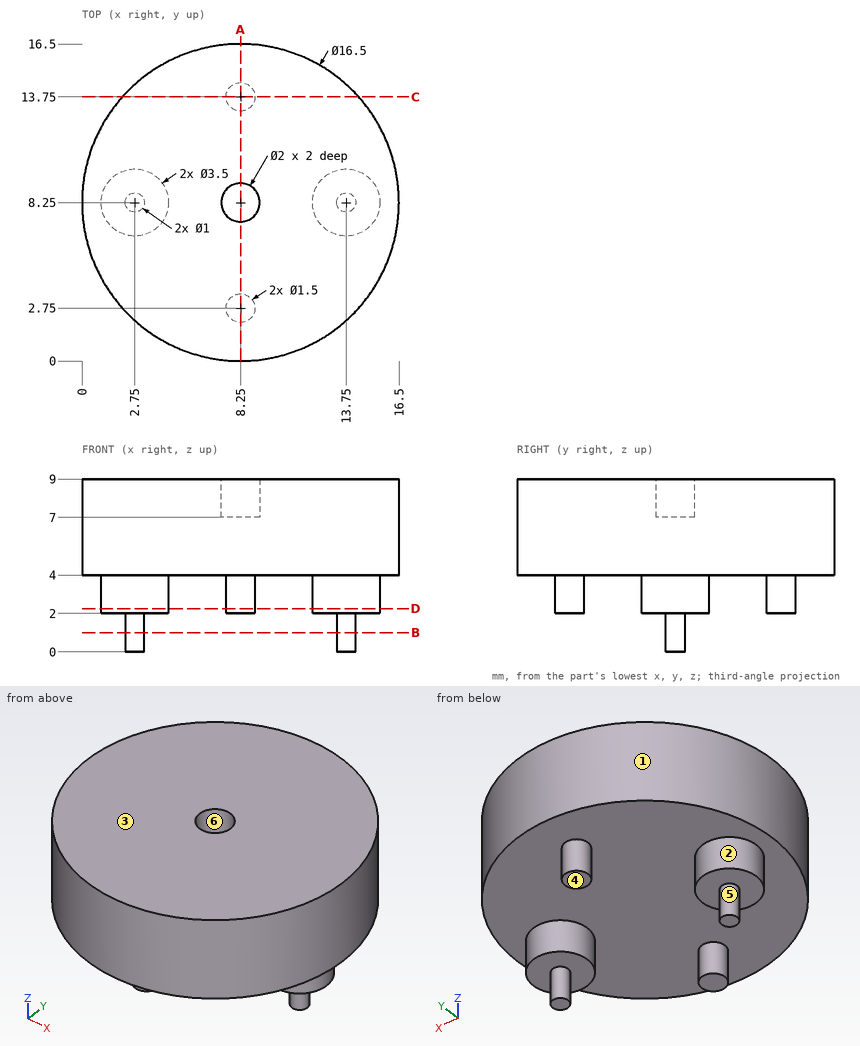
Input: dimensioned drawing with shaded views. Units: mm. Origin: part minimum x, y, z. A direction names the side the tool comes from. Coordinates: 2 decimals unless noted, no trailing zeros. Write each loop counter-clockwise with the first axis right and the second up, starting at its lowest first coordinate (ties: lowest second). Pieces come first, ordered by that corner, then holes. Notation, with made-up numbers: M -37.5,44.25 L -9.5,44.25 A19 cw -9.5,70.25 Z; hole C 38.25,1.25 d9. An arc over 180 degrees is marked long. Use one line per item in the form item = value.
Q1. Draft query along X for the marked faces 1, 2 and 3. Return one class per face: released by +X, released by -X, zero draft, split by the parting line, or undercut.
Answer below:
face_1 = split by the parting line
face_2 = undercut
face_3 = zero draft
Q2. Section B-B (z = 1). Return loops of the section in (x, y), plus the area to 3 significant figures.
Answer below:
outline = C 2.75,8.25 d1; C 13.75,8.25 d1
area = 1.57 mm²
Q3. Section A-A (x = 8.25). Return loops of the section in (y, z), plus the area to 3 significant figures.
Answer below:
outline = M 0,4 L 2,4 L 2,2 L 3.5,2 L 3.5,4 L 13,4 L 13,2 L 14.5,2 L 14.5,4 L 16.5,4 L 16.5,9 L 9.25,9 L 9.25,7 L 7.25,7 L 7.25,9 L 0,9 Z
area = 84.5 mm²
Q4. First-contact query: pin 1 (2 mm diameter, centred on y = 11, z = 3.5, fed in from -X); pin 2 (0.8 mm diameter, centred on x = 8.5, y = 2.5, fed in from -Z); pin 3 (1 mm diameter, centred on x = 2.5, y = 11, fed in from -Z). Flat tips, straight axial feed; report the tip coordinate or a pass-through.
Answer below:
pin_1 = 0.22
pin_2 = 2
pin_3 = 4
Q5. Section D-D (z = 2.25). Return loops of the section in (x, y), plus the area to 3 significant figures.
Answer below:
outline = C 2.75,8.25 d3.5; C 8.25,2.75 d1.5; C 8.25,13.75 d1.5; C 13.75,8.25 d3.5
area = 22.8 mm²
Q6. Set-up query: the marked faces 4, 5 and 6. Return all of +Z, -Z, +X, -X, +Y, -Y with unobstructed straight access to the full face (end or side cutting, diameter ignored); none if empty.
Answer below:
face_4 = -Z, +X, -X, +Y, -Y
face_5 = -Z
face_6 = +Z
Q7. Section C-C (y = 13.75). Return loops of the section in (x, z), plus the area to 3 significant figures.
Answer below:
outline = M 2.1,4 L 7.5,4 L 7.5,2 L 9,2 L 9,4 L 14.4,4 L 14.4,9 L 2.1,9 Z
area = 64.5 mm²
Q8. Material intervals for probe 1 along Y at (x, z) = (8.25, 8); probe 2 along Z at (x, y) = (9, 13.5); probe 3 along X at (y, z) = (8.75, 3.75), sorted ascending. Write a range as from..to.
Answer below:
probe_1 = 0..7.25, 9.25..16.5
probe_2 = 4..9
probe_3 = 1.07..4.43, 12.07..15.43
